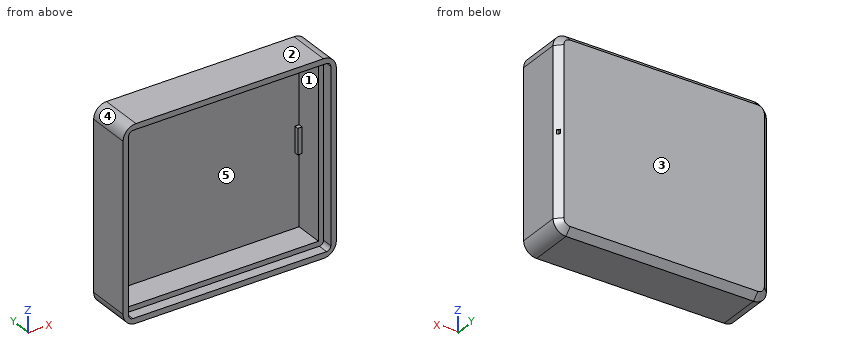
from build123d import *

# Parameters (mm, degrees)
SKETCH1_W           = 50
SKETCH1_H           = 11.666666667
BOSS_EXTRUDE1_DEPTH = 45
SKETCH2_W           = 1
SKETCH2_H           = 1
CUT_EXTRUDE1_DEPTH  = 1
SHELL1_T            = -2.5
SKETCH3_W           = 47.4
SKETCH3_H           = 42.4
SKETCH3_W_2         = 45
SKETCH3_H_2         = 40
CUT_EXTRUDE3_DEPTH  = 2.5
FILLET1_R           = 1
FILLET2_R           = 3
CHAMFER1_SIZE       = 1.5


with BuildPart() as part:
    # Sketch1 → Boss-Extrude1 (new body)
    with BuildSketch(Plane.XY):
        with Locations((25, 5.833333334)):
            Rectangle(SKETCH1_W, SKETCH1_H)
    extrude(amount=BOSS_EXTRUDE1_DEPTH)

    # Sketch2 → Cut-Extrude1 (cut)
    with BuildSketch(Plane(origin=(50, 0, 0), x_dir=(0, 0, -1), z_dir=(1, 0, 0))):
        with Locations((-22.5, 11.166666667)):
            Rectangle(SKETCH2_W, SKETCH2_H)
    extrude(amount=-CUT_EXTRUDE1_DEPTH, mode=Mode.SUBTRACT)

    # Shell1
    shell1_openings = [part.faces().sort_by_distance(p)[0] for p in [
        (25, 0, 22.5),
    ]]
    offset(amount=SHELL1_T, openings=shell1_openings, kind=Kind.INTERSECTION)

    # Sketch3 → Cut-Extrude3 (cut)
    with BuildSketch(Plane.XZ):
        with Locations((25, 22.5)):
            Rectangle(SKETCH3_W, SKETCH3_H)
        with Locations((25, 22.5)):
            Rectangle(SKETCH3_W_2, SKETCH3_H_2, mode=Mode.SUBTRACT)
    extrude(amount=-CUT_EXTRUDE3_DEPTH, mode=Mode.SUBTRACT)

    # Fillet1
    fillet1_edges = [part.edges().sort_by_distance(p)[0] for p in [
        (1.3, 1.25, 1.3),
        (1.3, 1.25, 43.7),
        (48.7, 1.25, 43.7),
        (48.7, 1.25, 1.3),
    ]]
    fillet(fillet1_edges, radius=FILLET1_R)

    # Fillet2
    fillet2_edges = [part.edges().sort_by_distance(p)[0] for p in [
        (50, 5.833333333, 45),
        (0, 5.833333333, 45),
        (50, 5.833333333, 0),
        (0, 5.833333333, 0),
    ]]
    fillet(fillet2_edges, radius=FILLET2_R)

    # Chamfer1
    # the kernel refuses this chamfer: 1.5 mm, written as the material it takes off along each edge
    with BuildSketch(Plane(origin=(50, 11.666666667, 19.142475518), x_dir=(0.027495876610586768, -0.9996219169112968, 0), z_dir=(0, 0, 1)), Plane(origin=(50, 11.666666667, 3), x_dir=(0.027495876610586768, -0.9996219169112968, 0), z_dir=(0, 0, 1))) as chamfer1_piece_1:
        Polygon((CHAMFER1_SIZE * 0.999621916911, -CHAMFER1_SIZE * 0.0274958766106), (-CHAMFER1_SIZE * 0.0274958766106, -CHAMFER1_SIZE * 0.999621916911), (0, 0), align=None)
    extrude(amount=22.857524482, mode=Mode.SUBTRACT)
    with BuildSketch(Plane(origin=(47, 11.666666667, 42), x_dir=(0, 0, 1), z_dir=(-1, 0, 0))) as chamfer1_piece_2:
        Polygon((3, -CHAMFER1_SIZE), (3 - CHAMFER1_SIZE, 0), (3, 0), align=None)
    revolve(axis=Axis((47, 11.666666667, 42), (0, 1, 0)), revolution_arc=90, mode=Mode.SUBTRACT)
    with BuildSketch(Plane(origin=(47, 11.666666667, 3), x_dir=(0, 0, -1), z_dir=(-1, 0, 0))) as chamfer1_piece_3:
        Polygon((3, CHAMFER1_SIZE), (3 - CHAMFER1_SIZE, 0), (3, 0), align=None)
    revolve(axis=Axis((47, 11.666666667, 3), (0, -1, 0)), revolution_arc=90, mode=Mode.SUBTRACT)
    with BuildSketch(Plane(origin=(47, 11.666666667, 45), x_dir=(0, -0.9996219169112965, 0.02749587661058676), z_dir=(-1, 0, 0))) as chamfer1_piece_4:
        Polygon((CHAMFER1_SIZE * 0.999621916911, -CHAMFER1_SIZE * 0.0274958766106), (-CHAMFER1_SIZE * 0.0274958766106, -CHAMFER1_SIZE * 0.999621916911), (0, 0), align=None)
    extrude(amount=44, mode=Mode.SUBTRACT)
    with BuildSketch(Plane(origin=(47, 11.666666667, 0), x_dir=(0, -0.9996219169112968, -0.02749587661058636), z_dir=(-1, 0, 0))) as chamfer1_piece_5:
        Polygon((CHAMFER1_SIZE * 0.999621916911, CHAMFER1_SIZE * 0.0274958766106), (-CHAMFER1_SIZE * 0.0274958766106, CHAMFER1_SIZE * 0.999621916911), (0, 0), align=None)
    extrude(amount=44, mode=Mode.SUBTRACT)
    with BuildSketch(Plane(origin=(3, 11.666666667, 42), x_dir=(-1, 0, 0), z_dir=(0, 0, -1))) as chamfer1_piece_6:
        Polygon((3, -CHAMFER1_SIZE), (3 - CHAMFER1_SIZE, 0), (3, 0), align=None)
    revolve(axis=Axis((3, 11.666666667, 42), (0, 1, 0)), revolution_arc=90, mode=Mode.SUBTRACT)
    with BuildSketch(Plane(origin=(3, 11.666666667, 3), x_dir=(-1, 0, 0), z_dir=(0, 0, 1))) as chamfer1_piece_7:
        Polygon((3, CHAMFER1_SIZE), (3 - CHAMFER1_SIZE, 0), (3, 0), align=None)
    revolve(axis=Axis((3, 11.666666667, 3), (0, -1, 0)), revolution_arc=90, mode=Mode.SUBTRACT)
    with BuildSketch(Plane(origin=(0, 11.666666667, 3), x_dir=(-0.02749587661058636, -0.9996219169112968, 0), z_dir=(0, 0, 1))) as chamfer1_piece_8:
        Polygon((CHAMFER1_SIZE * 0.999621916911, CHAMFER1_SIZE * 0.0274958766106), (-CHAMFER1_SIZE * 0.0274958766106, CHAMFER1_SIZE * 0.999621916911), (0, 0), align=None)
    extrude(amount=39, mode=Mode.SUBTRACT)


solid = part.part
Geometry: final body of the model. Coordinates: model frame, mm. Face numbers are marked on the shaded views. A direction names the side the tool comes from. Give positions to 0.01 mm unless a question says otherwise; leave off trailing zeros. Order: outer loops, then holes, each group sorted by start corner. A loop starts at its lowest first (then second) coordinate and runs counter-clockwise, first axis right, second up. Notation, with made-up numbers: (77, -36) - (109, -36) arc R20 cw to (109, -19) - close; hole circle Ø3 at (63.5, 80.25). An arc over 180 degrees is marked (long way). Use CSV: the item, a comma, the result in double quotes.
1. Contact query for flat-ended pins moving along their axis: pin 1 (2 mm diameter, centred on x = 14, z = 6, fed in from -Y); pin 2 (0.5 mm diameter, centred on x = 47, z = 21.5, fed in from -Y). Output: stop coordinate, or through.
Answers below:
pin 1,"y = 9.17"
pin 2,"y = 8.17"
2. Material intervals for line 1 along Z through (x, y) = (42, 1.5); line 2 along Z through (x, y) = (18, 3.25); line 3 along X through (y, z) = (6.5, 23), sorted ascending. Write a range as from..to.
Answers below:
line 1,"0..1.3, 43.7..45"
line 2,"0..2.5, 42.5..45"
line 3,"0..2.5, 47.5..50"
3. Section query B-B (z = 33). Output: boundary loops of the cut face in (x, y).
Answers below:
outline,"(0, 0) - (1.3, 0) - (1.3, 2.5) - (2.5, 2.5) - (2.5, 9.17) - (47.5, 9.17) - (47.5, 2.5) - (48.7, 2.5) - (48.7, 0) - (50, 0) - (50, 10.17) - (48.5, 11.67) - (1.5, 11.67) - (0, 10.17) - close"
4. Section query A-A (y = 7). Output: boundary loops of the cut face in (x, z), plus the area to 3 significant figures.
Answers below:
outline,"(0, 3) arc R3 ccw to (3, 0) - (47, 0) arc R3 ccw to (50, 3) - (50, 42) arc R3 ccw to (47, 45) - (3, 45) arc R3 ccw to (0, 42) - close; hole (2.5, 2.5) - (47.5, 2.5) - (47.5, 42.5) - (2.5, 42.5) - close"
area,"442 mm2"
5. Access query for the marked faces 1 and 2. Directions: +Z, -Z, +X, -X, +Y, -Y. A direction counts if a zero-diameter tool reaches every point of the face in a straight line with its end or side. Return the directions, or none.
Answers below:
face 1,"-Y"
face 2,"+Z, +X, -X, +Y, -Y"
6. Mould query, pull axis X, two halves, no side actions, for the marked faces 3, 4 and 5. Classes: +X half, -X half, draft (parallel to the pull), parting line (faces both ways), or undercut.
Answers below:
face 3,"draft"
face 4,"-X half"
face 5,"undercut"
7. Section query C-C (x = 30). Output: boundary loops of the cut face in (y, z).
Answers below:
outline,"(0, 0) - (10.17, 0) - (11.67, 1.5) - (11.67, 43.5) - (10.17, 45) - (0, 45) - (0, 43.7) - (2.5, 43.7) - (2.5, 42.5) - (9.17, 42.5) - (9.17, 2.5) - (2.5, 2.5) - (2.5, 1.3) - (0, 1.3) - close"
